Autodesk Inventor part; units mm, degrees
ref_plane "YZ Plane" through (0, 0, 0) normal (1, 0, 0) x (0, 1, 0)
ref_plane "XZ Plane" through (0, 0, 0) normal (0, 1, 0) x (-1, 0, 0)
ref_plane "XY Plane" through (0, 0, 0) normal (0, 0, 1) x (1, 0, 0)
sketch "Sketch1" plane through (0, 0, 0) normal (1, 0, 0) x (0, 1, 0)
  line L0 (0, 0) -> (0, 20)
  line L1 (0, 20) -> (-15, 20)
  line L2 (0, 0) -> (3, 0)
  line L3 (3, 0) -> (3, 23)
  line L4 (3, 23) -> (-12, 23)
  line L5 (-12, 23) -> (-12, 28)
  line L6 (-12, 28) -> (-15, 28)
  line L7 (-15, 28) -> (-15, 20)
  line L8 (3.6548, 0) -> (-1.246, 0)
  line L9 (0, 0) -> (0, -20)
  line L10 (0, -20) -> (-15, -20)
  line L11 (3, 0) -> (3, -23)
  line L12 (3, -23) -> (-12, -23)
  line L13 (-12, -23) -> (-12, -28)
  line L14 (-15, -28) -> (-15, -20)
  line L15 (-12, -28) -> (-15, -28)
  line L16 (-12, 28) -> (-12, 30)
  line L17 (-12, 30) -> (-15, 30)
  line L18 (-15, 30) -> (-15, 28)
  line L19 (-15, -28) -> (-15, -30)
  line L20 (-15, -30) -> (-12, -30)
  line L21 (-12, -30) -> (-12, -28)
  dimension "d0" = 20
  dimension "d1" = 15
  dimension "d2" = 3
  dimension "d3" = 23
  dimension "d4" = 15
  dimension "d5" = 5
  dimension "d22" = 2
  dimension "d23" = 2
extrude "Extrusion1" add sketch "Sketch1" along normal blind 7 and the other way blind 2
sketch "Sketch2" plane through (0, -12, 28) normal (0, 1, 0) x (1, 0, 0)
  line L0 (0, 0) -> (-2, 2.1)
  line L1 (-2, -2) -> (-2, 5)
  line L2 (-2, 58) -> (-2, 48)
  line L3 (0, 56) -> (-2, 54.5)
  point P0 (0, 28)
  point P1 (2.5, 2.5)
  point P2 (2.5, 53.5)
  dimension "d8" = 2.9
  dimension "d9" = 2.5
hole "Hole1" at (2.5, -12, 25.5) at (2.5, -12, -25.5) direction (0, -1, 0) diameter 3.4 end through all
sketch "Sketch3" plane through (0, -12, 28) normal (0, 1, 0) x (1, 0, 0)
  circle A0 centre (2.5, 2.5) radius 1.7
  circle A1 centre (2.5, 2.5) radius 3
  circle A2 centre (2.5, 53.5) radius 1.7
  circle A3 centre (2.5, 53.5) radius 3
  point P0 (0, 28)
  dimension "d17" = 6
  dimension "d18" = 6
fillet "Fillet1" radius 2 4 edges at (2.5, 3, 23) (2.5, 0, 20) (2.5, 0, -20) (2.5, 3, -23)
extrude "Extrusion2" cut sketch "Sketch3" along normal blind 20
properties part number "esc-bracket"
The model under review builds one solid part; all positions refer to its coordinate system, in mm. A direction names the side the tool comes from. Give positions to 0.01 mm unless a question says otherwise; leave off trailing zeros. Order: outer loops, then holes, each group sorted by start corner. A loop starts at its lowest first (then second) coordinate and runs counter-clockwise, first axis right, second up. Notation, with made-up numbers: M 56.25,29 L 101.25,29 A28 cw 101.25,57 Z; hole C -21,36.25 d7. An arc over 180 degrees is marked long. Use one line per item in the form item = value. Start each with the question number.
Item 1: We need section D-D on x = 6. Give the boundary of the cut face in (y, z), plus the area to 3 significant figures.
Item 2: To check wall thickness, follow line 1 along Z through (x, y) = (2.5, -13.25); line 2 along Z through (x, y) = (6, -7.5); line 3 along X through (y, z) = (-13.6, 25.5). State the ranges of each line that lie inside material, in increasing order. Write a range as from..to.
Item 3: We need section B-B on z = -25.5. Give the boundary of the cut face in (x, y), plus the area to 3 significant figures.
Item 4: The part is to be moulded in two halves that separate along X. For faces 6 (the flat face through (7, 1, 0)), 7 (the cylindrical face through (3.15, -13.52, -23.93)), 8 (the flat face through (2, -14, -30)), say which applies: pulls with the +X half, pulls with the -X half, needs draft (parallel to the pull), parting line crosses it, or undercut.
Item 5: We need section C-C on y = -7.75. Give the boundary of the cut face in (x, z).
Item 6: We need section A-A on x = 2.5. Give the boundary of the cut face in (y, z).
Item 7: For faces 1 (the cylindrical face through (2.5, -4.9, 22.5)), 2 (the cylindrical face through (2.5, -4.9, -22.5)), 3 (the flat face through (6, -5, 23)), 4 (the flat face through (2, -8, 20)), 5 (the flat face through (2, 3, 0)), list the 3-axis set-ups (+Z, -Z, +X, -X, +Y, -Y) from which the entire face can be reached by the end or side of a thin tool; tool diameter is ignored.
Item 8: Insertion check: pin 1 Ø3 at (x, y) = (3.5, -8) entering from +Z; pin 2 Ø2.5 at (x, y) = (0.5, -6) entering from -Z; pin 3 Ø1.5 at (x, z) = (4, 5) entering from -Y. Each pin has a flat end and moves straight along its axis. Give the tip position at first contact, or say it passes through.
Completed:
q1.outline = M -15,-30 L -12,-30 L -12,-23 L 1,-23 A2 ccw 3,-21 L 3,21 A2 ccw 1,23 L -12,23 L -12,30 L -15,30 L -15,20 L -2,20 A2 cw 0,18 L 0,-18 A2 cw -2,-20 L -15,-20 Z
q1.area = 270 mm²
q2.line_1 = -30..-27.2, -23.8..-20, 20..23.8, 27.2..30
q2.line_2 = -23..-20, 20..23
q2.line_3 = -2..0.8, 4.2..7
q3.outline = M -2,-15 L 0.8,-15 L 0.8,-12 L -2,-12 Z; M 4.2,-15 L 7,-15 L 7,-12 L 4.2,-12 Z
q3.area = 16.8 mm²
q4.face_6 = pulls with the +X half
q4.face_7 = undercut
q4.face_8 = needs draft
q5.outline = M -2,-23 L 0.84,-23 A3 cw 4.16,-23 L 7,-23 L 7,-20 L -2,-20 Z; M -2,20 L 7,20 L 7,23 L 4.16,23 A3 cw 0.84,23 L -2,23 Z
q6.outline = M -15,-30 L -12,-30 L -12,-27.2 L -15,-27.2 Z; M -15,-23.8 L -12,-23.8 L -12,-22.5 L 2.32,-22.5 A2 ccw 3,-21 L 3,21 A2 ccw 2.32,22.5 L -12,22.5 L -12,23.8 L -15,23.8 L -15,20 L -2,20 A2 cw 0,18 L 0,-18 A2 cw -2,-20 L -15,-20 Z; M -15,27.2 L -12,27.2 L -12,30 L -15,30 Z
q7.face_1 = +Z, +Y
q7.face_2 = -Z, +Y
q7.face_3 = +Z, +X, -X, +Y
q7.face_4 = +X, -X, -Y
q7.face_5 = +Z, -Z, +X, -X, +Y
q8.pin_1 = 23
q8.pin_2 = -23
q8.pin_3 = 0
